CAD build for the part. Positions are in the model's coordinates, mm. A direction names the side the tool comes from. Round coordinates to 2 decimals unless told otherwise and drop trailing zeros. Loops run counter-clockwise (first coordinate to the right, second up) from the corner with the lowest first, then second, coordinate; pieces in that order, holes last. Notation, with made-up numbers: (-8.75, 26.25) -> (22.25, 26.25) arc R28 cw to (22.25, 57.25) -> close; hole circle Ø10 at (67.25, 11.25). An arc over 180 degrees is marked (long way). Answer as CSV lines item,"result".
```python
from build123d import *

# Parameters (mm, degrees)
F0_W     = 8.255
F0_H     = 4.445
F1_DEPTH = 12.7


with BuildPart() as f1:
    # F0 (on Top) → F1 (new body)
    with BuildSketch(Plane.XY):
        with BuildLine():
            Line((3.175, 89.2175), (-3.175, 89.2175))
            Line((-3.175, 89.2175), (-3.175, 59.21375))
            ThreePointArc((-3.175, 59.21375), (-1.4603208006, 53.1557160458), (3.175, 48.895))
            Line((3.175, 48.895), (3.175, 54.3686230183))
            Line((3.175, 54.3686230183), (3.175, 89.2175))
        make_face()
        with BuildLine():
            ThreePointArc((3.175, 48.895), (-1.4603208006, 53.1557160458), (-3.175, 59.21375))
            Line((-3.175, 59.21375), (-3.175, 35.0967737428))
            ThreePointArc((-3.175, 35.0967737428), (-1.6043069816, 35.4435836373), (0, 35.56))
            ThreePointArc((0, 35.56), (1.6318769104, 35.751593167), (3.175, 36.315952381))
            Line((3.175, 36.315952381), (3.175, 48.895))
        make_face()
        with BuildLine():
            ThreePointArc((5.178111588, 52.8630686695), (4.1097442392, 53.5269543338), (3.175, 54.3686230183))
            Line((3.175, 54.3686230183), (3.175, 48.895))
            ThreePointArc((3.175, 48.895), (7.0454761905, 42.6054761905), (3.175, 36.315952381))
            Line((3.175, 36.315952381), (3.175, 31.5623598693))
            ThreePointArc((3.175, 31.5623598693), (11.4400029348, 41.5296621103), (5.178111588, 52.8630686695))
        make_face()
        with BuildLine():
            ThreePointArc((0, 35.56), (-1.6043069816, 35.4435836373), (-3.175, 35.0967737428))
            Line((-3.175, 35.0967737428), (-3.175, 30.3105138368))
            ThreePointArc((-3.175, 30.3105138368), (-1.6376677767, 30.9107499954), (0, 31.115))
            ThreePointArc((0, 31.115), (1.6031808891, 31.2273896149), (3.175, 31.5623598693))
            Line((3.175, 31.5623598693), (3.175, 36.315952381))
            ThreePointArc((3.175, 36.315952381), (1.6318769104, 35.751593167), (0, 35.56))
        make_face()
        with BuildLine():
            Line((-3.175, 30.3105138368), (-3.175, 35.0967737428))
            ThreePointArc((-3.175, 35.0967737428), (-11.1125, 24.4475), (-3.175, 13.7982262572))
            Line((-3.175, 13.7982262572), (-3.175, 18.5844861632))
            ThreePointArc((-3.175, 18.5844861632), (-6.6675, 24.4475), (-3.175, 30.3105138368))
        make_face()
        with BuildLine():
            ThreePointArc((0, 31.115), (-1.6376677767, 30.9107499954), (-3.175, 30.3105138368))
            Line((-3.175, 30.3105138368), (-3.175, 18.5844861632))
            ThreePointArc((-3.175, 18.5844861632), (-1.6376677767, 17.9842500046), (0, 17.78))
            ThreePointArc((0, 17.78), (1.6043069816, 17.6635836373), (3.175, 17.3167737428))
            Line((3.175, 17.3167737428), (3.175, 31.5623598693))
            ThreePointArc((3.175, 31.5623598693), (1.6031808891, 31.2273896149), (0, 31.115))
        make_face()
        with BuildLine():
            ThreePointArc((0, 13.335), (-1.6043069816, 13.4514163627), (-3.175, 13.7982262572))
            Line((-3.175, 13.7982262572), (-3.175, -0.4632262572))
            ThreePointArc((-3.175, -0.4632262572), (-1.6043069816, -0.1164163627), (0, 0))
            ThreePointArc((0, 0), (1.6376677767, 0.2042500046), (3.175, 0.8044861632))
            Line((3.175, 0.8044861632), (3.175, 12.5305138368))
            ThreePointArc((3.175, 12.5305138368), (1.6376677767, 13.1307499954), (0, 13.335))
        make_face()
        with BuildLine():
            Line((-3.175, 18.5844861632), (-3.175, 13.7982262572))
            ThreePointArc((-3.175, 13.7982262572), (-1.6043069816, 13.4514163627), (0, 13.335))
            ThreePointArc((0, 13.335), (1.6376677767, 13.1307499954), (3.175, 12.5305138368))
            Line((3.175, 12.5305138368), (3.175, 17.3167737428))
            ThreePointArc((3.175, 17.3167737428), (1.6043069816, 17.6635836373), (0, 17.78))
            ThreePointArc((0, 17.78), (-1.6376677767, 17.9842500046), (-3.175, 18.5844861632))
        make_face()
        with BuildLine():
            ThreePointArc((0, 0), (-1.6043069816, -0.1164163627), (-3.175, -0.4632262572))
            Line((-3.175, -0.4632262572), (-3.175, -5.2494861632))
            ThreePointArc((-3.175, -5.2494861632), (-1.6376677767, -4.6492500046), (0, -4.445))
            ThreePointArc((0, -4.445), (1.6043069816, -4.3285836373), (3.175, -3.9817737428))
            Line((3.175, -3.9817737428), (3.175, 0.8044861632))
            ThreePointArc((3.175, 0.8044861632), (1.6376677767, 0.2042500046), (0, 0))
        make_face()
        with BuildLine():
            Line((-3.175, -5.2494861632), (-3.175, -0.4632262572))
            ThreePointArc((-3.175, -0.4632262572), (-11.1125, -11.1125), (-3.175, -21.7617737428))
            Line((-3.175, -21.7617737428), (-3.175, -16.9755138368))
            ThreePointArc((-3.175, -16.9755138368), (-6.6675, -11.1125), (-3.175, -5.2494861632))
        make_face()
        with BuildLine():
            ThreePointArc((3.175, -3.9817737428), (11.1125, 6.6675), (3.175, 17.3167737428))
            Line((3.175, 17.3167737428), (3.175, 12.5305138368))
            ThreePointArc((3.175, 12.5305138368), (6.6675, 6.6675), (3.175, 0.8044861632))
            Line((3.175, 0.8044861632), (3.175, -3.9817737428))
        make_face()
        with BuildLine():
            ThreePointArc((0, -4.445), (-1.6376677767, -4.6492500046), (-3.175, -5.2494861632))
            Line((-3.175, -5.2494861632), (-3.175, -16.9755138368))
            ThreePointArc((-3.175, -16.9755138368), (-1.6376677767, -17.5757499954), (0, -17.78))
            ThreePointArc((0, -17.78), (1.6043069816, -17.8964163627), (3.175, -18.2432262572))
            Line((3.175, -18.2432262572), (3.175, -3.9817737428))
            ThreePointArc((3.175, -3.9817737428), (1.6043069816, -4.3285836373), (0, -4.445))
        make_face()
        with BuildLine():
            ThreePointArc((0, -22.225), (-1.6043069816, -22.1085836373), (-3.175, -21.7617737428))
            Line((-3.175, -21.7617737428), (-3.175, -36.0232262572))
            ThreePointArc((-3.175, -36.0232262572), (-1.6043069816, -35.6764163627), (0, -35.56))
            ThreePointArc((0, -35.56), (1.6376677767, -35.3557499954), (3.175, -34.7555138368))
            Line((3.175, -34.7555138368), (3.175, -23.0294861632))
            ThreePointArc((3.175, -23.0294861632), (1.6376677767, -22.4292500046), (0, -22.225))
        make_face()
        with BuildLine():
            Line((-3.175, -16.9755138368), (-3.175, -21.7617737428))
            ThreePointArc((-3.175, -21.7617737428), (-1.6043069816, -22.1085836373), (0, -22.225))
            ThreePointArc((0, -22.225), (1.6376677767, -22.4292500046), (3.175, -23.0294861632))
            Line((3.175, -23.0294861632), (3.175, -18.2432262572))
            ThreePointArc((3.175, -18.2432262572), (1.6043069816, -17.8964163627), (0, -17.78))
            ThreePointArc((0, -17.78), (-1.6376677767, -17.5757499954), (-3.175, -16.9755138368))
        make_face()
        with BuildLine():
            ThreePointArc((0, -35.56), (-1.6043069816, -35.6764163627), (-3.175, -36.0232262572))
            Line((-3.175, -36.0232262572), (-3.175, -40.8094861632))
            ThreePointArc((-3.175, -40.8094861632), (-1.6376677767, -40.2092500046), (0, -40.005))
            ThreePointArc((0, -40.005), (1.6043069816, -39.8885836373), (3.175, -39.5417737428))
            Line((3.175, -39.5417737428), (3.175, -34.7555138368))
            ThreePointArc((3.175, -34.7555138368), (1.6376677767, -35.3557499954), (0, -35.56))
        make_face()
        with BuildLine():
            Line((-3.175, -40.8094861632), (-3.175, -36.0232262572))
            ThreePointArc((-3.175, -36.0232262572), (-11.1125, -46.6725), (-3.175, -57.3217737428))
            Line((-3.175, -57.3217737428), (-3.175, -52.5355138368))
            ThreePointArc((-3.175, -52.5355138368), (-6.6675, -46.6725), (-3.175, -40.8094861632))
        make_face()
        with BuildLine():
            ThreePointArc((3.175, -39.5417737428), (11.1125, -28.8925), (3.175, -18.2432262572))
            Line((3.175, -18.2432262572), (3.175, -23.0294861632))
            ThreePointArc((3.175, -23.0294861632), (6.6675, -28.8925), (3.175, -34.7555138368))
            Line((3.175, -34.7555138368), (3.175, -39.5417737428))
        make_face()
        with BuildLine():
            ThreePointArc((0, -40.005), (-1.6376677767, -40.2092500046), (-3.175, -40.8094861632))
            Line((-3.175, -40.8094861632), (-3.175, -52.5355138368))
            ThreePointArc((-3.175, -52.5355138368), (-1.6376677767, -53.1357499954), (0, -53.34))
            Line((0, -53.34), (3.175, -53.34))
            Line((3.175, -53.34), (3.175, -39.5417737428))
            ThreePointArc((3.175, -39.5417737428), (1.6043069816, -39.8885836373), (0, -40.005))
        make_face()
        with BuildLine():
            ThreePointArc((0, -57.785), (-1.6043069816, -57.6685836373), (-3.175, -57.3217737428))
            Line((-3.175, -57.3217737428), (-3.175, -69.5325))
            Line((-3.175, -69.5325), (3.175, -69.5325))
            Line((3.175, -69.5325), (3.175, -57.785))
            Line((3.175, -57.785), (0, -57.785))
        make_face()
        with BuildLine():
            Line((-3.175, -52.5355138368), (-3.175, -57.3217737428))
            ThreePointArc((-3.175, -57.3217737428), (-1.6043069816, -57.6685836373), (0, -57.785))
            Line((0, -57.785), (3.175, -57.785))
            Line((3.175, -57.785), (3.175, -53.34))
            Line((3.175, -53.34), (0, -53.34))
            ThreePointArc((0, -53.34), (-1.6376677767, -53.1357499954), (-3.175, -52.5355138368))
        make_face()
        with Locations((7.3025, -55.5625)):
            Rectangle(F0_W, F0_H)
    extrude(amount=F1_DEPTH)


solid = f1.part
```
Q1. Slice it at B-B, the plane y = 4. Give the cut face in (x, z) (3 decimals).
Results:
outline,"(-3.175, 0) -> (3.175, 0) -> (3.175, 12.7) -> (-3.175, 12.7) -> close; (6.111, 0) -> (10.788, 0) -> (10.788, 12.7) -> (6.111, 12.7) -> close"
Q2. Tool access for faces 1 (the flat face through (3.175, -11, 6)), 2 (the flat face through (-3.175, -47, 6)), 3 (the flat face through (-3.175, 7, 6)): list every direction of +Z, -Z, +X, -X, +Y, -Y with a clear straight run to the whole face (end or side of a thin tool).
Results:
face 1,"+Z, -Z, +X"
face 2,"+Z, -Z"
face 3,"+Z, -Z, -X"
Q3. Slice it at D-D, the plane y = 74.5. Give the cut face in (x, z) (3 decimals), and give its area (3 significant figures).
Results:
outline,"(-3.175, 0) -> (3.175, 0) -> (3.175, 12.7) -> (-3.175, 12.7) -> close"
area,"80.6 mm2"
Q4. Slice it at A-A, the plane x = -4.75. Give the cut face in (y, z).
Results:
outline,"(-56.72, 0) -> (-51.35, 0) -> (-51.35, 12.7) -> (-56.72, 12.7) -> close; (-41.99, 0) -> (-36.63, 0) -> (-36.63, 12.7) -> (-41.99, 12.7) -> close; (-21.16, 0) -> (-15.79, 0) -> (-15.79, 12.7) -> (-21.16, 12.7) -> close; (-6.43, 0) -> (-1.07, 0) -> (-1.07, 12.7) -> (-6.43, 12.7) -> close; (14.4, 0) -> (19.77, 0) -> (19.77, 12.7) -> (14.4, 12.7) -> close; (29.13, 0) -> (34.49, 0) -> (34.49, 12.7) -> (29.13, 12.7) -> close"
Q5. Probe L1, parallel to Y at x = 7.5, z = 8.75 (3 decimals); L2, parallel to X at y = -29, z = 7.25 (3 decimals); L3, parallel to X at y = 42, z = 12.25 (3 decimals). List the from-to ranges inside material, lowest first. Write a range as [from, to].
Results:
L1,"[-57.785, -53.34], [-37.092, -20.693], [-1.532, 14.867], [33.9, 51.311]"
L2,"[-3.175, 3.175], [6.667, 11.112]"
L3,"[-3.175, 3.175], [7.019, 11.475]"
Q6. Slice it at C-C, the plane z = 6. Count the separate pieces of the cut face and the enclosed holes in it, and give its area (3 significant figures).
Results:
separate pieces,"1"
enclosed holes,"6"
area,"1,620 mm2"
Q7. Two-plate mould, pull along Y, no slides. Class faces 4 (the flat face through (0, 89.218, 6)), 5 (the cylindrical face through (11.42, 41.34, 6.26)), 6 (the flat face through (0, 11, 12.7)): pulls with the +Y half, pulls with the -Y half, needs draft (parallel to the pull), parting line crosses it, or undercut.
Results:
face 4,"pulls with the +Y half"
face 5,"undercut"
face 6,"needs draft"
Q8. Drop flat-ended pins along their axis: pin 1 Ø4 at (y, z) = (74.5, 6) entering from +X (3 decimals); pin 2 Ø4 at (y, z) = (3.5, 4) entering from -X (3 decimals); pin 3 Ø1.5 at (y, z) = (47, 3.5) entering from +X; pin 4 Ø1 at (x, y) = (9, 33) entering from -Z. Give the stop position or say it passes through.
Results:
pin 1,"x = 3.175"
pin 2,"x = -3.175"
pin 3,"x = 10.9"
pin 4,"through"
